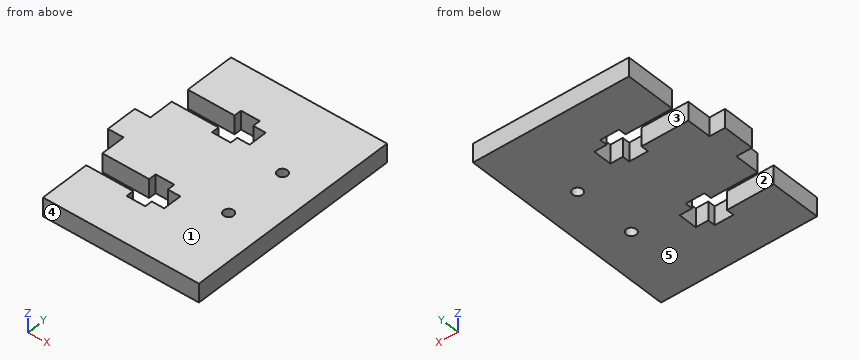
```python
from build123d import *

# Parameters (mm, degrees)
SKETCH1_R           = 1.6
BOSS_EXTRUDE1_DEPTH = 6


with BuildPart() as part:
    # Sketch1 → Boss-Extrude1 (new body)
    with BuildSketch(Plane.XY):
        Polygon((-121, -35), (-71, -35), (-71, 35), (-121, 35), (-121, 18.9), (-106, 18.9), (-106, 21.3), (-100, 21.3), (-100, 18.9), (-96, 18.9), (-96, 12.9), (-100, 12.9), (-100, 10.5), (-106, 10.5), (-106, 12.9), (-121, 12.9), (-121, 5), (-126, 5), (-126, -5), (-121, -5), (-121, -12.9), (-106, -12.9), (-106, -10.5), (-100, -10.5), (-100, -12.9), (-96, -12.9), (-96, -18.9), (-100, -18.9), (-100, -21.3), (-106, -21.3), (-106, -18.9), (-121, -18.9), align=None)
        with Locations((-83, -10)):
            Circle(SKETCH1_R, mode=Mode.SUBTRACT)
        with Locations((-83, 10)):
            Circle(SKETCH1_R, mode=Mode.SUBTRACT)
    extrude(amount=BOSS_EXTRUDE1_DEPTH)


solid = part.part
```
Geometry: final body of the model. Coordinates: model frame, mm. Face numbers are marked on the shaded views. A direction names the side the tool comes from. Coordinates: 2 decimals unless noted, no trailing zeros. Order: outer loops, then holes, each group sorted by start corner. A loop starts at its lowest first (then second) coordinate and runs counter-clockwise, first axis right, second up. Notation, with made-up numbers: (89, 76.5) -> (134, 76.5) arc R20 ccw to (134, 110.5) -> close; hole circle Ø4 at (4.25, 12). An arc over 180 degrees is marked (long way). Use CSV: the item, a comma, the result in double quotes.
1) Mould query, pull axis Y, two halves, no side actions, for the marked faces 3, 4 and 5. Classes: +Y half, -Y half, draft (parallel to the pull), parting line (faces both ways), or undercut.
Findings:
face 3,"undercut"
face 4,"-Y half"
face 5,"draft"
2) Section A-A on x = -83. Output: boundary loops of the cut face in (y, z), then the cut area to 3 significant figures.
Findings:
outline,"(-35, 0) -> (-11.6, 0) -> (-11.6, 6) -> (-35, 6) -> close; (-8.4, 0) -> (8.4, 0) -> (8.4, 6) -> (-8.4, 6) -> close; (11.6, 0) -> (35, 0) -> (35, 6) -> (11.6, 6) -> close"
area,"382 mm^2"
3) Line query: line 1 (Y direction, x = -83, z = 2.75); line 2 (Y direction, x = -102.5, z = 1.45); line 3 (X direction, y = -12.5, z = 1.6). Output: solid intervals per line, ascending.
Findings:
line 1,"y = -35 to -11.6, -8.4 to 8.4, 11.6 to 35"
line 2,"y = -35 to -21.3, -10.5 to 10.5, 21.3 to 35"
line 3,"x = -121 to -106, -100 to -71"
4) Section C-C on x = -115.5. Output: boundary loops of the cut face in (y, z), then the cut area to 3 significant figures.
Findings:
outline,"(-35, 0) -> (-18.9, 0) -> (-18.9, 6) -> (-35, 6) -> close; (-12.9, 0) -> (12.9, 0) -> (12.9, 6) -> (-12.9, 6) -> close; (18.9, 0) -> (35, 0) -> (35, 6) -> (18.9, 6) -> close"
area,"348 mm^2"
5) Section D-D on y = 23.5. Output: boundary loops of the cut face in (x, z).
Findings:
outline,"(-121, 0) -> (-71, 0) -> (-71, 6) -> (-121, 6) -> close"
6) Access query for the marked faces 1 and 2. Directions: +Z, -Z, +X, -X, +Y, -Y. A direction counts if a zero-diameter tool reaches every point of the face in a straight line with its end or side. Return the directions, or none.
Findings:
face 1,"+Z, +X, -X, +Y, -Y"
face 2,"+Z, -Z, -X"
7) Pin query (flat end, axial travel): pin 1 Ø2.5 at (x, y) = (-83, 10) entering from -Z; pin 2 Ø3 at (y, z) = (10, 2) entering from -X. Return the tip coordinate at first contact, or that it passes through.
Findings:
pin 1,"passes through"
pin 2,"stops at x = -121"
8) Section B-B on z = 5.15. State how many separate pieces and enclosed holes the cut face has, then the cut area to 3 significant figures.
Findings:
separate pieces,"1"
enclosed holes,"2"
area,"3,180 mm^2"
